Read the model definition and answer for the solid it produces. Units are mm, in the model's axes. A direction names the side the tool comes from. Coordinates: 2 decimals unless noted, no trailing zeros. Write each loop counter-clockwise with the first axis right and the second up, starting at its lowest first coordinate (ties: lowest second). Pieces come first, ordered by that corner, then holes.
Item 1: Each of these flat-tipped pins is pushed along its axis until it touches: P1, Ø6, axis at x = -50, y = 13.5, coming from the -Z side; P2, Ø8, axis at x = -48, z = 1.5, coming from the -Y side; P3, Ø10, axis at x = 3, z = -10.5, coming from the -Y side; P4, Ø6.5, axis at x = 50.8, y = 0, coming from the -Z side. Where does it stop, or does it pass through?
Item 2: Determine the mould class of faces 3 (the face through (2.75, -12.4, -17.53)), 4 (the face through (0, 6, -35.56)), 5 (the face through (0, 0, 0)) for opening direction X: released by +X, released by -X, zero draft, split by the parting line, or undercut.
Item 3: Section A-A (x = -50.8) is taken. Give the vertices of the cut face in (y, z), then the cut area to 3 significant figures.
Item 4: Section B-B (y = 0) is taken. Give the vertices of the cut face in (x, z).
Item 5: Straight lines are drawn through the part: probe 1 along Y at (x, z) = (0, -25); probe 2 along Z at (x, y) = (18, -43); probe 3 along X at (y, z) = (-7, -29.5). For each, find the intervals that lie inside material, in ascending order.
Item 6: Section D-D (z = -14.5) is taken. Give the vertices of the cut face in (x, y) (1 decimal).
Item 7: A tool of negligible diameter and unlimited length cuts with its end or side. For faces 1 (the face through (-0.72, -45.29, 6.26)), 2 (the face through (0, 5.064, -18)), from which of +Z, -Z, +X, -X, +Y, -Y can it reach the whole face along a straight path? Write none if from no direction.
from build123d import *

# Parameters (mm, degrees)
SKETCH1_R           = 63.5
SKETCH1_R_2         = 5.55625
BOSS_EXTRUDE1_DEPTH = 12.7
SKETCH2_R           = 12.7
BOSS_EXTRUDE2_DEPTH = 35.56


with BuildPart() as part:
    # Sketch1 → Boss-Extrude1 (new body)
    with BuildSketch(Plane.XY):
        Circle(SKETCH1_R)
        with Locations((-50.8, 0)):
            Circle(SKETCH1_R_2, mode=Mode.SUBTRACT)
        with Locations((0, 50.8)):
            Circle(SKETCH1_R_2, mode=Mode.SUBTRACT)
        with Locations((50.8, 0)):
            Circle(SKETCH1_R_2, mode=Mode.SUBTRACT)
        with Locations((0, -50.8)):
            Circle(SKETCH1_R_2, mode=Mode.SUBTRACT)
    extrude(amount=BOSS_EXTRUDE1_DEPTH)

    # Sketch2 → Boss-Extrude2 (add)
    with BuildSketch(Plane(origin=(0, 0, 0), x_dir=(-1, 0, 0), z_dir=(0, 0, -1))):
        Circle(SKETCH2_R)
        with BuildLine():
            Line((-2.3876, 7.569892502), (-2.3876, 5.063801502))
            Line((-2.3876, 5.063801502), (2.3876, 5.063801502))
            Line((2.3876, 5.063801502), (2.3876, 7.569892502))
            ThreePointArc((2.3876, 7.569892502), (0, -7.9375), (-2.3876, 7.569892502))
        make_face(mode=Mode.SUBTRACT)
    extrude(amount=BOSS_EXTRUDE2_DEPTH)


solid = part.part
Established:
1. P1: stops at z = 0
1. P2: stops at y = -45.78
1. P3: stops at y = -12.7
1. P4: passes through
2. face 3: split by the parting line
2. face 4: zero draft
2. face 5: undercut
3. outline: (-38.1, 0) - (-5.56, 0) - (-5.56, 12.7) - (-38.1, 12.7) - close; (5.56, 0) - (38.1, 0) - (38.1, 12.7) - (5.56, 12.7) - close
3. area: 827 mm2
4. outline: (-63.5, 0) - (-56.36, 0) - (-56.36, 12.7) - (-63.5, 12.7) - close; (-45.24, 0) - (-12.7, 0) - (-12.7, -35.56) - (-7.94, -35.56) - (-7.94, 0) - (7.94, 0) - (7.94, -35.56) - (12.7, -35.56) - (12.7, 0) - (45.24, 0) - (45.24, 12.7) - (-45.24, 12.7) - close; (56.36, 0) - (63.5, 0) - (63.5, 12.7) - (56.36, 12.7) - close
5. probe 1: y = -12.7 to -7.94, 5.06 to 12.7
5. probe 2: z = 0 to 12.7
5. probe 3: x = -10.6 to -3.74, 3.74 to 10.6
6. outline: circle Ø25.4 at (0, 0); hole (-2.4, 5.1) - (-2.4, 7.6) arc R7.9 ccw (long way) to (2.4, 7.6) - (2.4, 5.1) - close
7. face 1: +Z, -Z
7. face 2: -Z
